Geometry check sheet. Reference: the model listing, model coordinates, mm. A direction names the side the tool comes from. Round coordinates to 2 decimals unless told otherwise and drop trailing zeros. Write each loop counter-clockwise with the first axis right and the second up, starting at its lowest first coordinate (ties: lowest second). Pieces come first, ordered by that corner, then holes.
Autodesk Fusion 360 part; units mm, degrees
sketch "Sketch1" plane through (0, 0, 0) normal (0, 0, 1) x (1, 0, 0)
  line L0 (0, 0) -> (30.5, 0)
  line L1 (30.5, 0) -> (30.5, 70)
  line L2 (30.5, 70) -> (0, 70)
  line L3 (0, 70) -> (0, 0)
  line L4 (0, 35) -> (30.5, 35) construction
  line L5 (15.25, 70) -> (15.25, 0) construction
  line L6 (0, 0) -> (9, 0)
  line L7 (9, 0) -> (9, 6)
  line L8 (6, 9) -> (0, 9)
  line L9 (0, 9) -> (0, 0)
  arc A0 (9, 6) -> (6, 9) centre (6, 6) ccw
  line L10 (21.5, 0) -> (21.5, 6)
  arc A1 (24.5, 9) -> (21.5, 6) centre (24.5, 6) ccw
  line L11 (24.5, 9) -> (30.5, 9)
  line L12 (9, 70) -> (9, 64)
  arc A2 (6, 61) -> (9, 64) centre (6, 64) ccw
  line L13 (6, 61) -> (0, 61)
  line L14 (21.5, 70) -> (21.5, 64)
  arc A3 (21.5, 64) -> (24.5, 61) centre (24.5, 64) ccw
  line L15 (24.5, 61) -> (30.5, 61)
  point P0 (15.25, 35)
  dimension "d1" = 70
  dimension "d2" = 30.5
  dimension "d3" = 15.25
  dimension "d4" = 35
  dimension "d5" = 9
  dimension "d6" = 9
  dimension "d7" = 3
extrude "Extrude1" add sketch "Sketch1" along normal blind 17 contours L0 L1 L2 L3 L7 L8 A0 L10 A1 L11 L12 A2 L13 L14 A3 L15
ref_plane "WorkPlane1" through (15.25, 35, 16) normal (0, 0, 1) x (1, 0, 0)
sketch "Sketch2" plane through (15.25, 35, 16) normal (0, 0, 1) x (1, 0, 0)
  line L0 (15.25, 35) -> (-15.25, 35)
  line L1 (-15.25, 35) -> (-15.25, -35)
  line L2 (-15.25, -35) -> (15.25, -35)
  line L3 (15.25, -35) -> (15.25, 35)
  line L4 (15.25, 35) -> (-15.25, -35) construction
  line L5 (-15.25, 35) -> (15.25, -35) construction
  circle A0 centre (-12.25, 32) radius 1.75
  line L6 (0, 35) -> (0, -35) construction
  line L7 (-15.25, 0) -> (15.25, 0) construction
  circle A1 centre (12.25, 32) radius 1.75
  circle A2 centre (-12.25, -32) radius 1.75
  circle A3 centre (12.25, -32) radius 1.75
  dimension "d13" = 30.5
  dimension "d14" = 70
  dimension "d33" = 3.5
  dimension "d34" = 12.25
  dimension "d35" = 32
extrude "Extrude2" add sketch "Sketch2" against normal blind 1.5
sketch "Sketch4" plane through (0, 0, 0) normal (0, 0, -1) x (-1, 0, 0)
  line L0 (-9, 70) -> (-21.5, 70)
  line L1 (-21.5, 70) -> (-21.5, 64)
  arc A0 (-24.5, 61) -> (-21.5, 64) centre (-24.5, 64) ccw
  line L2 (-24.5, 61) -> (-30.5, 61)
  line L3 (-30.5, 61) -> (-30.5, 9)
  line L4 (-30.5, 9) -> (-24.5, 9)
  arc A1 (-21.5, 6) -> (-24.5, 9) centre (-24.5, 6) ccw
  line L5 (-21.5, 6) -> (-21.5, 0)
  line L6 (-21.5, 0) -> (-9, 0)
  line L7 (-9, 0) -> (-9, 6)
  arc A2 (-6, 9) -> (-9, 6) centre (-6, 6) ccw
  line L8 (-6, 9) -> (0, 9)
  line L9 (0, 9) -> (0, 61)
  line L10 (0, 61) -> (-6, 61)
  arc A3 (-9, 64) -> (-6, 61) centre (-6, 64) ccw
  line L11 (-9, 64) -> (-9, 70)
  line L12 (-21.5, 70) -> (-9, 70)
  line L13 (-9, 70) -> (-9, 67)
  line L14 (-9, 67) -> (-21.5, 67)
  line L15 (-21.5, 67) -> (-21.5, 70)
  line L16 (-21.5, 0) -> (-9, 0)
  line L17 (-9, 0) -> (-9, 2)
  line L18 (-9, 2) -> (-21.5, 2)
  line L19 (-21.5, 2) -> (-21.5, 0)
  dimension "d19" = 3
  dimension "d20" = 12.5
  dimension "d21" = 2
extrude "Extrude3" cut sketch "Sketch4" against normal up to surface (14.5 mm away) contours L0 L1 L11 L12 L13 L14 L15 | L5 L6 L7 L16 L17 L18 L19
sketch "Sketch5" plane through (0, 0, 17) normal (0, 0, 1) x (1, 0, 0)
  line L0 (21.5, 70) -> (9, 70)
  line L1 (9, 70) -> (9, 64)
  arc A0 (6, 61) -> (9, 64) centre (6, 64) ccw
  line L2 (6, 61) -> (0, 61)
  line L3 (0, 61) -> (0, 9)
  line L4 (0, 9) -> (6, 9)
  arc A1 (9, 6) -> (6, 9) centre (6, 6) ccw
  line L5 (9, 6) -> (9, 0)
  line L6 (9, 0) -> (21.5, 0)
  line L7 (21.5, 0) -> (21.5, 6)
  arc A2 (24.5, 9) -> (21.5, 6) centre (24.5, 6) ccw
  line L8 (24.5, 9) -> (30.5, 9)
  line L9 (30.5, 9) -> (30.5, 61)
  line L10 (30.5, 61) -> (24.5, 61)
  arc A3 (21.5, 64) -> (24.5, 61) centre (24.5, 64) ccw
  line L11 (21.5, 64) -> (21.5, 70)
  line L12 (29, 25.75) -> (29, 36.75)
  arc A4 (29, 36.75) -> (1.5, 36.75) centre (15.25, 36.75) ccw
  line L13 (1.5, 36.75) -> (1.5, 25.75)
  arc A5 (1.5, 25.75) -> (29, 25.75) centre (15.25, 25.75) ccw
  line L14 (15.25, 25.75) -> (15.25, 36.75) construction
  dimension "d27" = 27.5
  dimension "d28" = 11
  dimension "d29" = 25.75
  dimension "d30" = 15.25
extrude "Extrude4" cut sketch "Sketch5" against normal blind 2 contours L12 A4 L13 A5
sketch "Sketch6" plane through (0, 67, 0) normal (0, 1, 0) x (-1, 0, 0)
  line L0 (-9, 14.5) -> (-21.5, 14.5)
  line L1 (-21.5, 14.5) -> (-21.5, 0)
  line L2 (-21.5, 0) -> (-9, 0)
  line L3 (-9, 0) -> (-9, 14.5)
  line L4 (-11.25, 5) -> (-19.25, 5)
  line L5 (-19.25, 5) -> (-19.25, 2)
  line L6 (-19.25, 2) -> (-11.25, 2)
  line L7 (-11.25, 2) -> (-11.25, 5)
  line L8 (-11.25, 5) -> (-19.25, 2) construction
  line L9 (-19.25, 5) -> (-11.25, 2) construction
  point P0 (-15.25, 3.5)
  dimension "d39" = 3
  dimension "d40" = 8
  dimension "d41" = 2
  dimension "d43" = 15.25
extrude "Extrude5" cut sketch "Sketch6" against normal blind 10 contours L4 L5 L6 L7
fillet "Fillet3" radius 0.5 4 edges at (30.5, 70, 15.25) (0, 70, 15.25) (0, 0, 15.25) (30.5, 0, 15.25)
fillet "Fillet3" radius 0.5 16 edges at (0, 9, 7.25) (0, 9, 16.5) (9, 0, 16.5) (9, 2, 7.25) (21.5, 2, 7.25) (21.5, 0, 16.5) (30.5, 9, 16.5) (30.5, 9, 7.25) (30.5, 61, 16.5) (30.5, 61, 7.25) (21.5, 67, 7.25) (21.5, 70, 16.5) (9, 70, 16.5) (9, 67, 7.25) (0, 61, 7.25) (0, 61, 16.5)
fillet "Fillet3" radius 0.5 16 edges at (27.5, 61, 17) (22.3787, 61.8787, 17) (21.5, 67, 17) (9, 67, 17) (8.1213, 61.8787, 17) (3, 61, 17) (15.25, 70, 17) (0, 35, 17) (3, 9, 17) (8.1213, 8.1213, 17) (9, 3, 17) (15.25, 0, 17) (21.5, 3, 17) (22.3787, 8.1213, 17) (27.5, 9, 17) (30.5, 35, 17) 1 faces at (18.0516, 43.7072, 0)
equation "d28 = 38.5 mm - 27.5 mm"
equation "d29 = 12 mm + ( ( 27.5 / 2 ) * 1 mm )"
equation "d30 = ( 30.5 / 2 ) * 1 mm"
equation "d34 = ( ( 21 + 3.5 ) / 2 ) * 1 mm"
equation "d35 = ( ( 60.5 + 3.5 ) / 2 ) * 1 mm"
equation "d43 = ( 30.5 / 2 ) * 1 mm"
1. Section check B-B (x = 3). Record the cut outline in (y, z) (3 decimals), plus the area to 3 significant figures.
2. Scan lines: line 1 along X through (y, z) = (67, 15.45); line 2 along Y through (x, z) = (3, 14.9); line 3 along Y through (x, z) = (3, 15.25) (3 decimals). Record each from-to range of solid material in increasing order.
3. Section check A-A (y = 58). Record the cut outline in (x, z), plus the area to 3 significant figures.
4. Section check C-C (x = 15.25). Record the cut outline in (y, z), plus the area to 3 significant figures.
5. Section check D-D (y = 28). Record the cut outline in (x, z), plus the area to 3 significant figures.
6. Depth check by flat-ended pin: pin 1 Ø4.5 at (x, z) = (2.5, 6.5) entering from -Y; pin 2 Ø10.5 at (x, y) = (27, 6.5) entering from +Z; pin 3 Ø8 at (x, z) = (16, 9.5) entering from -Y; pin 4 Ø2 at (y, z) = (65.5, 7) entering from -X. Enter the tip coordinate at first touch or a pass-through.
7. Access from +Z, -Z, +X, -X, +Y, -Y to the whole of each face (thin tool, end or side, straight path). Record for faces 1 (the face through (8.14, 61.9, 7.4)), 2 (the face through (27, 61, 7)), 3 (the face through (26, 5, 16)), 4 (the face through (14.948, 12.003, 16.014)), 5 (the face through (19.25, 62, 4)).
8. Release check for a two-part mould opening along Y. For faces 6 (the face through (8.1, 8.14, 7.4)), 7 (the face through (22.4, 61.86, 7.4)), 8 (the face through (25.75, 3.08, 15.26)) record: +Y half, -Y half, draft (parallel to the pull), parting line (faces both ways), or undercut.
Results below:
1. outline: (0, 14.5) - (1.25, 14.5) - (1.25, 16) - (0, 16) - close; (4.75, 14.5) - (9, 14.5) - (9, 0.5) arc R0.5 ccw to (9.5, 0) - (60.5, 0) arc R0.5 ccw to (61, 0.5) - (61, 14.5) - (65.25, 14.5) - (65.25, 16) - (61, 16) - (61, 16.5) arc R0.5 ccw to (60.5, 17) - (42.995, 17) - (42.995, 15) - (19.505, 15) - (19.505, 17) - (9.5, 17) arc R0.5 ccw to (9, 16.5) - (9, 16) - (4.75, 16) - close; (68.75, 14.5) - (70, 14.5) - (70, 16) - (68.75, 16) - close
1. area: 853 mm2
2. line 1: x = 0 to 1.25, 4.75 to 25.75, 29.25 to 30.5
2. line 2: y = 0 to 1.25, 4.75 to 65.25, 68.75 to 70
2. line 3: y = 0 to 1.25, 4.75 to 19.505, 42.995 to 65.25, 68.75 to 70
3. outline: (0, 0.5) arc R0.5 ccw to (0.5, 0) - (30, 0) arc R0.5 ccw to (30.5, 0.5) - (30.5, 16.5) arc R0.5 ccw to (30, 17) - (0.5, 17) arc R0.5 ccw to (0, 16.5) - close; hole (11.25, 2) - (19.25, 2) - (19.25, 5) - (11.25, 5) - close
3. area: 494 mm2
4. outline: (0, 14.5) - (2, 14.5) - (2, 0.5) arc R0.5 ccw to (2.5, 0) - (66.5, 0) arc R0.5 ccw to (67, 0.5) - (67, 2) - (57, 2) - (57, 5) - (67, 5) - (67, 14.5) - (70, 14.5) - (70, 16.5) arc R0.5 ccw to (69.5, 17) - (50.5, 17) - (50.5, 15) - (12, 15) - (12, 17) - (0.5, 17) arc R0.5 ccw to (0, 16.5) - close
4. area: 1,010 mm2
5. outline: (0, 0.5) arc R0.5 ccw to (0.5, 0) - (30, 0) arc R0.5 ccw to (30.5, 0.5) - (30.5, 16.5) arc R0.5 ccw to (30, 17) - (29, 17) - (29, 15) - (1.5, 15) - (1.5, 17) - (0.5, 17) arc R0.5 ccw to (0, 16.5) - close
5. area: 463 mm2
6. pin 1: stops at y = 9
6. pin 2: stops at z = 17
6. pin 3: stops at y = 2
6. pin 4: stops at x = 9
7. face 1: -Z, -X, +Y
7. face 2: -Z, +X, +Y
7. face 3: +Z, +X, -Y
7. face 4: +Z
7. face 5: +Y
8. face 6: -Y half
8. face 7: +Y half
8. face 8: undercut
